Autodesk Inventor part; units mm, degrees
ref_plane "YZ Plane" through (0, 0, 0) normal (1, 0, 0) x (0, 1, 0)
ref_plane "XZ Plane" through (0, 0, 0) normal (0, 1, 0) x (-1, 0, 0)
ref_plane "XY Plane" through (0, 0, 0) normal (0, 0, 1) x (1, 0, 0)
sketch "Sketch1" plane through (0, 0, 0) normal (0, 1, 0) x (-1, 0, 0)
  line L0 (-62.5, -225.7) -> (62.5, -225.7)
  line L1 (62.5, -225.7) -> (62.5, 225.7)
  line L2 (62.5, 225.7) -> (-62.5, 225.7)
  line L3 (-62.5, 225.7) -> (-62.5, -225.7)
  line L4 (-62.5, -225.7) -> (62.5, 225.7) construction
  line L5 (62.5, -225.7) -> (-62.5, 225.7) construction
  point P0 (0, 0)
  dimension "d0" = 451.4
  dimension "d1" = 125
extrude "Extrusion1" add sketch "Sketch1" along normal blind 9.525
sketch "Sketch2" plane through (0, 9.525, 0) normal (0, 1, 0) x (1, 0, 0)
  line L0 (-62.5, 225.7) -> (-62.5, -225.7)
  line L1 (-62.5, -225.7) -> (-11.7, -225.7)
  line L2 (-11.7, -225.7) -> (-11.7, -200.3)
  line L3 (-11.7, -200.3) -> (-62.5, -200.3)
  line L4 (-62.5, -200.3) -> (-62.5, -225.7)
  line L5 (-62.5, 225.7) -> (-11.7, 225.7)
  line L6 (-11.7, 225.7) -> (-11.7, 200.3)
  line L7 (-11.7, 200.3) -> (-62.5, 200.3)
  line L8 (-62.5, 200.3) -> (-62.5, 225.7)
  point P0 (0, 0)
  point P1 (-62.5, 200.3)
  dimension "d4" = 25.4
  dimension "d5" = 25.4
  dimension "d6" = 50.8
  dimension "d7" = 50.8
extrude "Extrusion2" cut sketch "Sketch2" against normal through all
sketch "Sketch3" plane through (0, 0, 0) normal (0, 1, 0) x (1, 0, 0)
  line L0 (-62.5, 200.3) -> (-62.5, -200.3)
  line L1 (62.5, -225.7) -> (62.5, 225.7)
  point P0 (0, 0)
  point P1 (-47.5, 127)
  point P2 (47.7, -127)
  dimension "d10" = 254
  dimension "d11" = 95.2
  dimension "d12" = 127
  dimension "d13" = 15
  dimension "d14" = 14.8
hole "Hole1" at (-47.5, 0, -127) at (47.7, 0, 127) direction (0, 1, 0) diameter 9 end through all countersink diameter 17.3 countersink angle 90
equation "\"d5\" = d4"
equation "\"d7\" = d6"
properties part number "Shelf V1" material "Acetal Resin, Black"
Model file for the job. Use its own axes, mm. A direction names the side the tool comes from. Coordinates: 2 decimals unless noted, no trailing zeros. Order: outer loops, then holes, each group sorted by start corner. A loop starts at its lowest first (then second) coordinate and runs counter-clockwise, first axis right, second up. Notation, with made-up numbers: (79.5, 50.5) -> (103.5, 50.5) arc R18 cw to (103.5, 79.5) -> close; hole circle Ø8 at (29, 29.5). An arc over 180 degrees is marked (long way). Return JSON: item names as keys, results as strings. Group by question number.
Item 1: Saw through at A-A on z = -127. Write the cut outline in (x, y) (3 decimals), then the cut area to 3 significant figures.
Item 2: Saw through at C-C on y = 7.25. Write the cut outline in (x, z).
Item 3: Saw through at B-B on x = -47.5. Write the cut outline in (y, z) (3 decimals).
Item 4: Flat gauge pins, fed straight in: P1, Ø8, axis at x = 47.7, z = 127, coming from the +Y side; P2, Ø3, axis at x = -17.5, y = 7, coming from the -Z side; P3, Ø3, axis at y = 4, z = 215.5, coming from the -X side; P4, Ø5, axis at x = -48.5, y = 2.5, coming from the +Z side. Where does each tip first touch, or does it go through?
Item 5: Wall check: line 1 along X through (y, z) = (8.3, -127); line 2 along Z through (x, y) = (-47.5, 7.4); line 3 along X through (y, z) = (7.2, 127). Give the ranges that are in metal, low to high. Write a range as [from, to].
Item 6: Pull direction Z, two halves, no side cores. Call faces 4 (the cylindrical face through (-44.8, 6.9, -123.4)), 5 (the conical face through (44.804, 3.89, 130.777)), 6 (the flat face through (1, 9.525, 3)), 7 (the flat face through (26, 5, -225.7)): pulls with the +Z half, pulls with the -Z half, needs draft (parallel to the pull), parting line crosses it, or undercut.
Item 7: Tool access for faces 1 (the flat face through (-37, 5, -200.3)), 2 (the flat face through (-37, 5, 200.3)), 3 (the cylindrical face through (44.66, 6.88, 130.32)): list every direction of +Z, -Z, +X, -X, +Y, -Y with a clear straight run to the whole face (end or side of a thin tool).
Values found:
{
 "1": {"outline": "(-62.5, 0) -> (-56.15, 0) -> (-52, 4.15) -> (-52, 9.525) -> (-62.5, 9.525) -> close; (-43, 4.15) -> (-38.85, 0) -> (62.5, 0) -> (62.5, 9.525) -> (-43, 9.525) -> close", "area": "1,090 mm2"},
 "2": {"outline": "(-62.5, -200.3) -> (-11.7, -200.3) -> (-11.7, -225.7) -> (62.5, -225.7) -> (62.5, 225.7) -> (-11.7, 225.7) -> (-11.7, 200.3) -> (-62.5, 200.3) -> close; hole circle Ø9 at (-47.5, -127); hole circle Ø9 at (47.7, 127)"},
 "3": {"outline": "(0, -200.3) -> (9.525, -200.3) -> (9.525, -131.5) -> (4.15, -131.5) -> (0, -135.65) -> close; (0, -118.35) -> (4.15, -122.5) -> (9.525, -122.5) -> (9.525, 200.3) -> (0, 200.3) -> close"},
 "4": {"P1": "passes through", "P2": "stops at z = -200.3", "P3": "stops at x = -11.7", "P4": "stops at z = 200.3"},
 "5": {"line 1": "x = [-62.5, -52], [-43, 62.5]", "line 2": "z = [-200.3, -131.5], [-122.5, 200.3]", "line 3": "x = [-62.5, 43.2], [52.2, 62.5]"},
 "6": {"face 4": "undercut", "face 5": "undercut", "face 6": "needs draft", "face 7": "pulls with the -Z half"},
 "7": {"face 1": "-Z, -X, +Y, -Y", "face 2": "+Z, -X, +Y, -Y", "face 3": "+Y, -Y"}
}
